Part model, mm, in its own coordinate system. A direction names the side the tool comes from. Coordinates: 2 decimals unless noted, no trailing zeros. Write each loop counter-clockwise with the first axis right and the second up, starting at its lowest first coordinate (ties: lowest second). Pieces come first, ordered by that corner, then holes. Notation, with made-up numbers: (77.25, 47.25) - (82.25, 47.25) arc R24 cw to (82.25, 62.25) - close; hole circle Ø5 at (37, 6). An arc over 180 degrees is marked (long way). Use a Markdown table: item, result.
```python
from build123d import *

# Parameters (mm, degrees)
SKETCH1_R           = 12.7
BOSS_EXTRUDE1_DEPTH = 3
CUT_EXTRUDE1_DEPTH  = 10
SKETCH3_R           = 2
CUT_EXTRUDE2_DEPTH  = 5


with BuildPart() as part:
    # Sketch1 → Boss-Extrude1 (new body)
    with BuildSketch(Plane(origin=(0, 0, 0), x_dir=(1, 0, 0), z_dir=(0, 1, 0))):
        with Locations(Location((0, 0, 0), (0, 0, 270))):
            Circle(SKETCH1_R)
    extrude(amount=BOSS_EXTRUDE1_DEPTH)

    # Sketch2 → Cut-Extrude1 (cut)
    with BuildSketch(Plane(origin=(0, 3, 0), x_dir=(1, 0, 0), z_dir=(0, 1, 0))):
        with BuildLine():
            Line((2.765935685, -1.161722767), (1.956504764, 2.274222748))
            ThreePointArc((1.956504764, 2.274222748), (-2.92006701, -0.687901633), (2.765935685, -1.161722767))
        make_face()
    extrude(amount=-CUT_EXTRUDE1_DEPTH, mode=Mode.SUBTRACT)

    # Sketch3 → Cut-Extrude2 (cut)
    with BuildSketch(Plane(origin=(0, 3, 0), x_dir=(1, 0, 0), z_dir=(0, 1, 0))):
        with Locations(Location((0, 7, 0), (0, 0, 270))):
            Circle(SKETCH3_R)
        with Locations(Location((6.062177826, -3.5, 0), (0, 0, 270))):
            Circle(SKETCH3_R)
        with Locations(Location((-6.062177826, -3.5, 0), (0, 0, 270))):
            Circle(SKETCH3_R)
    extrude(amount=-CUT_EXTRUDE2_DEPTH, mode=Mode.SUBTRACT)


solid = part.part
```
Item 1: Band-saw the part on A-A, the plane x = 0. Give the cut face in (y, z), then the cut area to 3 significant figures.
From the geometry:
| item | result |
|---|---|
| outline | (0, -12.7) - (3, -12.7) - (3, -9) - (0, -9) - close; (0, -5) - (3, -5) - (3, -3) - (0, -3) - close; (0, 3) - (3, 3) - (3, 12.7) - (0, 12.7) - close |
| area | 46.2 mm^2 |
Item 2: Band-saw the part on B-B, the plane z = -7. Give the cut face in (x, y).
From the geometry:
| item | result |
|---|---|
| outline | (-10.6, 0) - (-2, 0) - (-2, 3) - (-10.6, 3) - close; (2, 0) - (10.6, 0) - (10.6, 3) - (2, 3) - close |
Item 3: Drop a flat-ended pin along its axis: P1, Ø1, axis at y = 1, z = -7.5, coming from the +X side. Give the stop position or say it passes through.
From the geometry:
| item | result |
|---|---|
| P1 | x = 10.6 |
Item 4: Band-saw the part on D-D, the plane z = -0.5. Give the cut face in (x, y).
From the geometry:
| item | result |
|---|---|
| outline | (-12.69, 0) - (-2.96, 0) - (-2.96, 3) - (-12.69, 3) - close; (2.37, 0) - (12.69, 0) - (12.69, 3) - (2.37, 3) - close |
Item 5: Drill centre lines: probe 1 along X at (y, z) = (1.35, 3.5); probe 2 along Z at (x, y) = (-1.75, 1.55); probe 3 along X at (y, z) = (0.8, 4.75). Where is each one in solid material? Low to high.
From the geometry:
| item | result |
|---|---|
| probe 1 | -12.21 to -8.06, -4.06 to 4.06, 8.06 to 12.21 |
| probe 2 | -12.58 to -7.97, -6.03 to -2.44, 2.44 to 12.58 |
| probe 3 | -11.78 to -7.62, -4.5 to 4.5, 7.62 to 11.78 |
Item 6: Two-plate mould, pull along Z, no slides. Class faces 1 (the face through (3, 3, 0)), 2 (the face through (-7.7, 1.5, -10.1)), 3 (the face through (-2.942, 1.521, 0.585)): pulls with the +Z half, pulls with the -Z half, needs draft (parallel to the pull), parting line crosses it, or undercut.
From the geometry:
| item | result |
|---|---|
| face 1 | needs draft |
| face 2 | parting line crosses it |
| face 3 | undercut |
Item 7: Which spindle directions (+Z, -Z, +X, -X, +Y, -Y) get a long thin tool onto all of the face, cutting with end or side? Do faces 4 (the face through (2.367, 1.521, -0.532)), 5 (the face through (3, 0, 0)). Say none if no direction does.
From the geometry:
| item | result |
|---|---|
| face 4 | +Y, -Y |
| face 5 | +Z, -Z, +X, -X, -Y |
Item 8: Band-saw the part on C-C, the plane y = 0.45. Give the cut face in (x, z).
From the geometry:
| item | result |
|---|---|
| outline | circle Ø25.4 at (0, 0); hole circle Ø4 at (-6.06, 3.5); hole circle Ø4 at (0, -7); hole (1.96, -2.27) - (2.77, 1.16) arc R3 ccw (long way) to start; hole circle Ø4 at (6.06, 3.5) |
